from build123d import *

# Parameters (mm, degrees)
EXTRUSION1_DEPTH        = 20
ENL_V_MAT_EXTRU_1_DEPTH = 300
ENL_V_MAT_EXTRU_3_DEPTH = 300
ENL_V_MAT_EXTRU_4_DEPTH = 21
ENL_V_MAT_EXTRU_7_DEPTH = 21


with BuildPart() as part:
    # Esquisse1 → Extrusion1 (new body)
    with BuildSketch(Plane.XY):
        with BuildLine():
            Line((-10, 8), (-10, -8))
            ThreePointArc((-10, -8), (-9.414213562, -9.414213562), (-8, -10))
            Line((-8, -10), (8, -10))
            ThreePointArc((8, -10), (9.414213562, -9.414213562), (10, -8))
            Line((10, -8), (10, 8))
            ThreePointArc((10, 8), (9.414213562, 9.414213562), (8, 10))
            Line((8, 10), (-8, 10))
            ThreePointArc((-8, 10), (-9.414213562, 9.414213562), (-10, 8))
        make_face()
    extrude(amount=EXTRUSION1_DEPTH)

    # Esquisse3 → Enlèv. mat.-Extru.1 (cut)
    with BuildSketch(Plane.XY.offset(20)):
        Polygon((10, 2.5), (8.2, 2.5), (8.2, 6), (3.7, 2.5), (3.7, -2.5), (8.2, -6), (8.2, -2.5), (10, -2.5), align=None)
    extrude(amount=-ENL_V_MAT_EXTRU_1_DEPTH, mode=Mode.SUBTRACT)

    # Esquisse5 → Enlèv. mat.-Extru.3 (cut)
    with BuildSketch(Plane.XY.offset(20)):
        Polygon((-2.5, 10), (-2.5, 8.2), (-6, 8.2), (-2.5, 3.7), (2.5, 3.7), (6, 8.2), (2.5, 8.2), (2.5, 10), align=None)
    extrude(amount=-ENL_V_MAT_EXTRU_3_DEPTH, mode=Mode.SUBTRACT)

    # Esquisse6 → Enlèv. mat.-Extru.4 (cut, through all)
    with BuildSketch(Plane.XY.offset(20)):
        Polygon((-2.5, -10), (-2.5, -8.2), (-6, -8.2), (-2.5, -3.7), (2.5, -3.7), (6, -8.2), (2.5, -8.2), (2.5, -10), align=None)
    extrude(amount=-ENL_V_MAT_EXTRU_4_DEPTH, mode=Mode.SUBTRACT)

    # Esquisse4 → Enlèv. mat.-Extru.7 (cut, through all)
    with BuildSketch(Plane.XY.offset(20)):
        Polygon((-10, 2.5), (-8.2, 2.5), (-8.2, 6), (-3.7, 2.5), (-3.7, -2.5), (-8.2, -6), (-8.2, -2.5), (-10, -2.5), align=None)
    extrude(amount=-ENL_V_MAT_EXTRU_7_DEPTH, mode=Mode.SUBTRACT)


solid = part.part
Verification items for the finished model (mm, model axes). A direction names the side the tool comes from. Give positions to 0.01 mm unless a question says otherwise; leave off trailing zeros. Order: outer loops, then holes, each group sorted by start corner. A loop starts at its lowest first (then second) coordinate and runs counter-clockwise, first axis right, second up. Notation, with made-up numbers: M -7,-19 L 23,-19 A26 ccw 23,6 Z; hole C 23,60.25 d7. An arc over 180 degrees is marked long. Answer as a JSON object with one key per item and string values. Group by question number.
1) Depth check by flat-ended pin: pin 1 Ø0.9 at (y, z) = (9, 9) entering from +X; pin 2 Ø1.5 at (x, z) = (-0.5, 6) entering from -Y; pin 3 Ø0.9 at (y, z) = (-9, 10) entering from -X. Enter the tip coordinate at first touch or a pass-through.
2) Cross-section at B-B (x = 4.5). Enter the section's corners in (y, z).
3) Mould release check, pull along Y, two halves, no side actions. Record for faces 1 (the face through (8.2, -4, 10)), 2 (the face through (-2.5, -9, 10)), 3 (the face through (9.43, 9.4, 9.86)), 4 (the face through (8.2, 4, 10)): released by +Y, released by -Y, zero draft, split by the parting line, or undercut.
4) Cross-section at C-C (x = 8.5). Enter the section's corners in (y, z).
5) Scan lines: line 1 along X through (y, z) = (2, 15); line 2 along Y through (x, z) = (5.75, 3); line 3 along Y through (x, z) = (3, 13.25). Record each from-to range of solid material in increasing order. Write a range as [from, to].
6) Cross-section at A-A (y = -3). Enter the section's corners in (x, z).
7) Access from +Z, -Z, +X, -X, +Y, -Y to the whole of each face (thin tool, end or side, straight path). Record for faces 5 (the face through (-9, -2.5, 10)), 6 (the face through (-2.5, 9, 10)), 7 (the face through (-5.919, -4.226, 10.14)).
8) Cross-section at D-D (y = -5). Enter the section's corners in (x, z), then the cut area to 3 significant figures.
Result sheet:
{
 "1": {"pin 1": "stops at x = 9.92", "pin 2": "stops at y = -3.7", "pin 3": "stops at x = -9.92"},
 "2": {"outline": "M -10,0 L -8.2,0 L -8.2,20 L -10,20 Z; M -6.27,0 L -3.12,0 L -3.12,20 L -6.27,20 Z; M 3.12,0 L 6.27,0 L 6.27,20 L 3.12,20 Z; M 8.2,0 L 10,0 L 10,20 L 8.2,20 Z"},
 "3": {"face 1": "undercut", "face 2": "zero draft", "face 3": "released by +Y", "face 4": "undercut"},
 "4": {"outline": "M -9.94,0 L -2.5,0 L -2.5,20 L -9.94,20 Z; M 2.5,0 L 9.94,0 L 9.94,20 L 2.5,20 Z"},
 "5": {"line 1": "x = [-3.7, 3.7]", "line 2": "y = [-10, -8.2], [-7.88, -4.09], [4.09, 7.88], [8.2, 10]", "line 3": "y = [-10, -8.2], [-4.34, 4.34], [8.2, 10]"},
 "6": {"outline": "M -10,0 L -8.2,0 L -8.2,20 L -10,20 Z; M -4.34,0 L 4.34,0 L 4.34,20 L -4.34,20 Z; M 8.2,0 L 10,0 L 10,20 L 8.2,20 Z"},
 "7": {"face 5": "+Z, -Z, -X", "face 6": "+Z, -Z, +Y", "face 7": "+Z, -Z"},
 "8": {"outline": "M -10,0 L -8.2,0 L -8.2,20 L -10,20 Z; M -6.91,0 L -3.51,0 L -3.51,20 L -6.91,20 Z; M 3.51,0 L 6.91,0 L 6.91,20 L 3.51,20 Z; M 8.2,0 L 10,0 L 10,20 L 8.2,20 Z", "area": "208 mm2"}
}
